Design review of the part built by this model. Coordinates are the model's own, in mm. Coordinates: 2 decimals unless noted, no trailing zeros. Loops run counter-clockwise (first coordinate to the right, second up) from the corner with the lowest first, then second, coordinate; pieces in that order, holes last. Notation, with made-up numbers: (61, -21) - (67, -21) arc R21 ccw to (67, 5) - close; hole circle Ø8 at (56.25, 54.25). An arc over 180 degrees is marked (long way). Answer in a Markdown table with one row per item. Add a question column.
(1) We need section A-A, the plane z = 87. Write out the cut boundary in (x, y), plus the area to 3 significant figures.
(2) To check wall thickness, follow L1, parallel to Z at x = -13.5, y = -26; L2, parallel to Z at x = -11.75, y = 14; L3, parallel to Y at x = -3.75, z = 52. State the ranges of each line that lie inside material, in increasing order. Write a range as [from, to].
(3) We need section B-B, the plane y = 3. Write out the cut boundary in (x, z).
(4) We need section C-C, the plane x = -6.5. Give the number of separate pieces and of enclosed holes in the cut face, plus the area to 3 significant figures.
(5) We need section D-D, the plane z = -72.5. Write out the cut boundary in (x, y).
(6) Clearance check with a flat-ended pin moving along its axis: pin 1 (6 mm diameter, centred on y = 40.31, z = -9.04, fed in from -X). State where the tip first meets the part, or that it passes through.
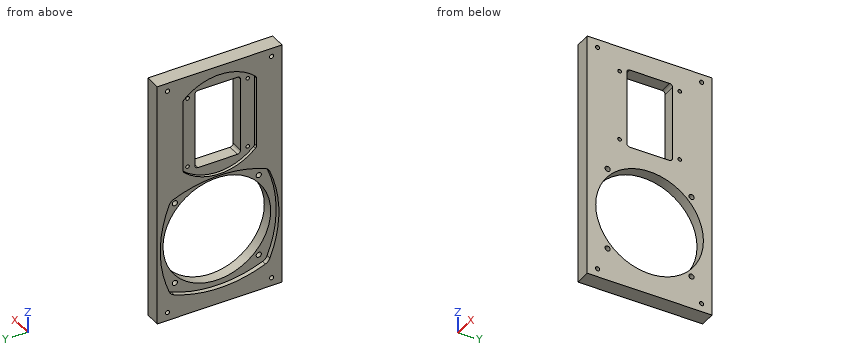
from build123d import *

# Parameters (mm, degrees)
F0_W     = 120
F0_H     = 240
F0_R     = 2
F0_R_2   = 1.75
F1_DEPTH = 15
F2_DEPTH = 12
F0_R_3   = 2.5
F0_R_4   = 51.75
F3_DEPTH = 10.5


with BuildPart() as f1:
    # F0 (on Right) → F1 (new body)
    with BuildSketch(Plane.YZ):
        with Locations((0, -1.592548)):
            Rectangle(F0_W, F0_H)
        with Locations((-49.999997, -113.592548)):
            Circle(F0_R, mode=Mode.SUBTRACT)
        with BuildLine():
            ThreePointArc((-43.965421, -1.013646), (0, 7.657452), (43.965421, -1.013646))
            ThreePointArc((43.965421, -1.013646), (46.58482, -2.757728), (48.328902, -5.377127))
            ThreePointArc((48.328902, -5.377127), (57, -49.342548), (48.328902, -93.307969))
            ThreePointArc((48.328902, -93.307969), (46.58482, -95.927368), (43.965421, -97.67145))
            ThreePointArc((43.965421, -97.67145), (0, -106.342548), (-43.965421, -97.67145))
            ThreePointArc((-43.965421, -97.67145), (-46.58482, -95.927368), (-48.328902, -93.307969))
            ThreePointArc((-48.328902, -93.307969), (-57, -49.342548), (-48.328902, -5.377127))
            ThreePointArc((-48.328902, -5.377127), (-46.58482, -2.757728), (-43.965421, -1.013646))
        make_face(mode=Mode.SUBTRACT)
        with Locations((50.000003, -113.592548)):
            Circle(F0_R, mode=Mode.SUBTRACT)
        with Locations((-45.415495, 59.40745)):
            Circle(F0_R_2, mode=Mode.SUBTRACT)
        with Locations((-49.999997, 110.407452)):
            Circle(F0_R, mode=Mode.SUBTRACT)
        with BuildLine():
            ThreePointArc((-34.517993, 95.849841), (-0.330971, 109.655772), (34.077245, 96.410744))
            ThreePointArc((34.077245, 96.410744), (34.794286, 95.408017), (35.047553, 94.201592))
            Line((35.047553, 94.201592), (35.047553, 24.613312))
            ThreePointArc((35.047553, 24.613312), (34.794286, 23.406887), (34.077245, 22.40416))
            ThreePointArc((34.077245, 22.40416), (-0.330971, 9.159132), (-34.517993, 22.965063))
            ThreePointArc((-34.517993, 22.965063), (-35.208951, 23.956802), (-35.452447, 25.140728))
            Line((-35.452447, 25.140728), (-35.452447, 93.674176))
            ThreePointArc((-35.452447, 93.674176), (-35.208951, 94.858102), (-34.517993, 95.849841))
        make_face(mode=Mode.SUBTRACT)
        with Locations((45.292415, 59.40745)):
            Circle(F0_R_2, mode=Mode.SUBTRACT)
        with Locations((50.000003, 110.407455)):
            Circle(F0_R, mode=Mode.SUBTRACT)
        with Locations((45.292415, 59.40745)):
            Circle(F0_R_2)
        with Locations((-45.415495, 59.40745)):
            Circle(F0_R_2)
    extrude(amount=-F1_DEPTH)

    # F0 (on Right) → F2 (join)
    with BuildSketch(Plane.YZ):
        with BuildLine():
            ThreePointArc((35.047553, 94.201592), (34.794286, 95.408017), (34.077245, 96.410744))
            ThreePointArc((34.077245, 96.410744), (-0.330971, 109.655772), (-34.517993, 95.849841))
            ThreePointArc((-34.517993, 95.849841), (-35.208951, 94.858102), (-35.452447, 93.674176))
            Line((-35.452447, 93.674176), (-35.452447, 25.140728))
            ThreePointArc((-35.452447, 25.140728), (-35.208951, 23.956802), (-34.517993, 22.965063))
            ThreePointArc((-34.517993, 22.965063), (-0.330971, 9.159132), (34.077245, 22.40416))
            ThreePointArc((34.077245, 22.40416), (34.794286, 23.406887), (35.047553, 24.613312))
            Line((35.047553, 24.613312), (35.047553, 94.201592))
        make_face()
        with Locations((-28.845534, 24.935452)):
            Circle(F0_R_2, mode=Mode.SUBTRACT)
        with Locations((-28.845534, 93.879452)):
            Circle(F0_R_2, mode=Mode.SUBTRACT)
        with Locations((29.005351, 24.935452)):
            Circle(F0_R_2, mode=Mode.SUBTRACT)
        with BuildLine():
            Line((-18.920092, 98.407452), (19.079908, 98.407452))
            ThreePointArc((19.079908, 98.407452), (21.201229, 97.528772), (22.079908, 95.407452))
            Line((22.079908, 95.407452), (22.079908, 23.407452))
            ThreePointArc((22.079908, 23.407452), (21.201229, 21.286132), (19.079908, 20.407452))
            Line((19.079908, 20.407452), (-18.920092, 20.407452))
            ThreePointArc((-18.920092, 20.407452), (-21.041412, 21.286132), (-21.920092, 23.407452))
            Line((-21.920092, 23.407452), (-21.920092, 95.407452))
            ThreePointArc((-21.920092, 95.407452), (-21.041412, 97.528772), (-18.920092, 98.407452))
        make_face(mode=Mode.SUBTRACT)
        with Locations((29.005351, 93.879452)):
            Circle(F0_R_2, mode=Mode.SUBTRACT)
    extrude(amount=-F2_DEPTH)

    # F0 (on Right) → F3 (join)
    with BuildSketch(Plane.YZ):
        with BuildLine():
            ThreePointArc((48.328902, -5.377127), (46.58482, -2.757728), (43.965421, -1.013646))
            ThreePointArc((43.965421, -1.013646), (0, 7.657452), (-43.965421, -1.013646))
            ThreePointArc((-43.965421, -1.013646), (-46.58482, -2.757728), (-48.328902, -5.377127))
            ThreePointArc((-48.328902, -5.377127), (-57, -49.342548), (-48.328902, -93.307969))
            ThreePointArc((-48.328902, -93.307969), (-46.58482, -95.927368), (-43.965421, -97.67145))
            ThreePointArc((-43.965421, -97.67145), (0, -106.342548), (43.965421, -97.67145))
            ThreePointArc((43.965421, -97.67145), (46.58482, -95.927368), (48.328902, -93.307969))
            ThreePointArc((48.328902, -93.307969), (57, -49.342548), (48.328902, -5.377127))
        make_face()
        with Locations((-40.305087, -89.647635)):
            Circle(F0_R_3, mode=Mode.SUBTRACT)
        with Locations((-40.305087, -9.037462)):
            Circle(F0_R_3, mode=Mode.SUBTRACT)
        with Locations((40.305087, -89.647635)):
            Circle(F0_R_3, mode=Mode.SUBTRACT)
        with Locations((0, -49.342548)):
            Circle(F0_R_4, mode=Mode.SUBTRACT)
        with Locations((40.305087, -9.037462)):
            Circle(F0_R_3, mode=Mode.SUBTRACT)
    extrude(amount=-F3_DEPTH)


solid = f1.part
Responses:
| question | item | result |
|---|---|---|
| 1 | outline | (-15, -60) - (0, -60) - (0, -21.92) - (-12, -21.92) - (-12, -35.45) - (-15, -35.45) - close; (-15, 35.05) - (-12, 35.05) - (-12, 22.08) - (0, 22.08) - (0, 60) - (-15, 60) - close |
| 1 | area | 1,060 mm2 |
| 2 | L1 | z = [-121.59, -103.39], [4.7, 16.46], [102.36, 118.41] |
| 2 | L2 | z = [-121.59, -105.49], [6.81, 20.41], [98.41, 118.41] |
| 2 | L3 | y = [-60, -21.92], [22.08, 60] |
| 3 | outline | (-15, -121.59) - (0, -121.59) - (0, -101.01) - (-10.5, -101.01) - (-10.5, -106.3) - (-15, -106.3) - close; (-15, 7.62) - (-10.5, 7.62) - (-10.5, 2.32) - (0, 2.32) - (0, 20.41) - (-12, 20.41) - (-12, 9.24) - (-15, 9.24) - close; (-15, 109.57) - (-12, 109.57) - (-12, 98.41) - (0, 98.41) - (0, 118.41) - (-15, 118.41) - close |
| 4 | separate pieces | 1 |
| 4 | enclosed holes | 14 |
| 4 | area | 16,800 mm2 |
| 5 | outline | (-15, -60) - (0, -60) - (0, -46.28) - (-10.5, -46.28) - (-10.5, -54.66) - (-15, -54.66) - close; (-15, 54.66) - (-10.5, 54.66) - (-10.5, 46.28) - (0, 46.28) - (0, 60) - (-15, 60) - close |
| 6 | pin 1 | stops at x = -10.5 |
